Work out the finished part from the listing and answer in its coordinate system (mm). A direction names the side the tool comes from. Coordinates: 2 decimals unless noted, no trailing zeros. Order: outer loops, then holes, each group sorted by start corner. A loop starts at its lowest first (then second) coordinate and runs counter-clockwise, first axis right, second up. Notation, with made-up numbers: (61.25, 10) -> (106.25, 10) arc R27 cw to (106.25, 38) -> close; hole circle Ø10 at (7, 22.25). An arc over 180 degrees is marked (long way). Answer as CSV lines item,"result". Start each with the question number.
Item 1: Straight lines are drawn through the part: L1, parallel to Z at x = 44, y = 12; L2, parallel to Z at x = 0, y = -10; L3, parallel to X at y = 8, z = 2.5. For each, find the intervals that lie inside material, in ascending order.
Item 2: Section A-A (y = 12.7) is taken. Write down the section's boundary in (x, z).
Item 3: Section D-D (x = 44) is taken. Write down the section's boundary in (y, z) (3 decimals).
Item 4: Which of the six approach directions +Z, -Z, +X, -X, +Y, -Y give full straight-line access (tool end or side, diameter ignored) to faces 4 (the face through (1.4, 11.112, 18.2)), 5 (the face through (8.2, -4.763, -8.2)), 6 (the face through (31.75, -13, -16)), 7 (the face through (25, 0, 25.4))?
Item 5: Section C-C (x = 6) is taken. Write down the section's boundary in (y, z) (1 decimal), then the cut area to 3 significant figures.
Item 6: Each of these flat-tipped pins is pushed along its axis until it touches: pin 1 Ø2.5 at (x, z) = (10.78, -10.78) entering from -Y; pin 2 Ø4 at (x, y) = (-5, 13) entering from -Z; pin 3 Ø8 at (x, y) = (-11.5, -2) entering from +Z; pin 4 Ø2 at (x, z) = (-10.78, -10.78) entering from -Y. Where does it stop, or does it pass through?
Item 7: For a pull along Y with two mould halves and no side action, classify faces 1 (the face through (-15.12, -13.62, -11.59)), 2 (the face through (31.75, 13, 16)), 3 (the face through (21, 22.225, 0)) as pulls with the +Y half, pulls with the -Y half, needs draft (parallel to the pull), parting line crosses it, or undercut.
```python
from build123d import *

# Parameters (mm, degrees)
SKETCH1_W           = 76.2
SKETCH1_H           = 50.8
BOSS_EXTRUDE1_DEPTH = 22.225
SKETCH2_R           = 20.5994
CUT_EXTRUDE1_DEPTH  = 11.1125
SKETCH3_R           = 18.0975
CUT_EXTRUDE2_DEPTH  = 9.525
SKETCH4_R           = 9.6266
CUT_EXTRUDE3_DEPTH  = 24.8125
SKETCH5_R           = 19.05
CUT_EXTRUDE4_DEPTH  = 17.4625
SKETCH6_R           = 11.303
CUT_EXTRUDE5_DEPTH  = 1.397
SKETCH7_R           = 3.2639
CUT_EXTRUDE6_DEPTH  = 19.05
SKETCH8_R           = 1.1811
CUT_EXTRUDE7_DEPTH  = 27.9875
CIRPATTERN1_COUNT   = 4
CUT_EXTRUDE8_DEPTH  = 45.45


with BuildPart() as part:
    # Sketch1 → Boss-Extrude1 (new body, symmetric)
    with BuildSketch(Plane(origin=(0, 0, 0), x_dir=(1, 0, 0), z_dir=(0, 1, 0))):
        with Locations((12.7, 0)):
            Rectangle(SKETCH1_W, SKETCH1_H)
    extrude(amount=BOSS_EXTRUDE1_DEPTH, both=True)

    # Sketch2 → Cut-Extrude1 (cut)
    with BuildSketch(Plane(origin=(0, 22.225, 0), x_dir=(1, 0, 0), z_dir=(0, 1, 0))):
        Circle(SKETCH2_R)
    extrude(amount=-CUT_EXTRUDE1_DEPTH, mode=Mode.SUBTRACT)

    # Sketch3 → Cut-Extrude2 (cut)
    with BuildSketch(Plane(origin=(0, 11.1125, 0), x_dir=(1, 0, 0), z_dir=(0, 1, 0))):
        Circle(SKETCH3_R)
    extrude(amount=-CUT_EXTRUDE2_DEPTH, mode=Mode.SUBTRACT)

    # Sketch4 → Cut-Extrude3 (cut, through all)
    with BuildSketch(Plane(origin=(0, 1.5875, 0), x_dir=(1, 0, 0), z_dir=(0, 1, 0))):
        Circle(SKETCH4_R)
    extrude(amount=-CUT_EXTRUDE3_DEPTH, mode=Mode.SUBTRACT)

    # Sketch5 → Cut-Extrude4 (cut)
    with BuildSketch(Plane.XZ.offset(22.225)):
        Circle(SKETCH5_R)
    extrude(amount=-CUT_EXTRUDE4_DEPTH, mode=Mode.SUBTRACT)

    # Sketch6 → Cut-Extrude5 (cut)
    with BuildSketch(Plane.XZ.offset(4.7625)):
        Circle(SKETCH6_R)
    extrude(amount=-CUT_EXTRUDE5_DEPTH, mode=Mode.SUBTRACT)

    # Sketch7 → Cut-Extrude6 (cut)
    with BuildSketch(Plane(origin=(50.8, 0, 0), x_dir=(0, 0, -1), z_dir=(1, 0, 0))):
        with Locations((-15.875, 12.7)):
            Circle(SKETCH7_R)
        with Locations((15.875, 12.7)):
            Circle(SKETCH7_R)
        with Locations((-15.875, -12.7)):
            Circle(SKETCH7_R)
        with Locations((15.875, -12.7)):
            Circle(SKETCH7_R)
    extrude(amount=-CUT_EXTRUDE6_DEPTH, mode=Mode.SUBTRACT)

    # Sketch8 → Cut-Extrude7 (cut, through all)
    with BuildSketch(Plane.XZ.offset(4.7625)):
        with Locations((-10.776307345, 10.776307345)):
            Circle(SKETCH8_R)
    cut_extrude7 = extrude(amount=-CUT_EXTRUDE7_DEPTH, mode=Mode.SUBTRACT)

    # CirPattern1: Cut-Extrude7 ×4 about axis
    cirpattern1_axis = Axis((0, 0, 0), (0, 1, 0))
    for i in range(1, CIRPATTERN1_COUNT):
        add(cut_extrude7.rotate(cirpattern1_axis, i * 360 / CIRPATTERN1_COUNT), mode=Mode.SUBTRACT)

    # Sketch9 → Cut-Extrude8 (cut, through all)
    with BuildSketch(Plane.XZ.offset(22.225)):
        with BuildLine():
            Line((0, 25.4), (0, 38.1))
            Line((0, 38.1), (-38.1, 38.1))
            Line((-38.1, 38.1), (-38.1, -38.1))
            Line((-38.1, -38.1), (0, -38.1))
            Line((0, -38.1), (0, -25.4))
            ThreePointArc((0, -25.4), (-25.4, 0), (0, 25.4))
        make_face()
    extrude(amount=-CUT_EXTRUDE8_DEPTH, mode=Mode.SUBTRACT)


solid = part.part
```
Checked values:
1,L1,"z = -25.4 to -19.06, -12.69 to 12.69, 19.06 to 25.4"
1,L2,"z = -25.4 to -19.05, 19.05 to 25.4"
1,L3,"x = -25.28 to -17.92, 17.92 to 50.8"
2,outline,"(0, -25.4) -> (50.8, -25.4) -> (50.8, -19.14) -> (31.75, -19.14) -> (31.75, -12.61) -> (50.8, -12.61) -> (50.8, 12.61) -> (31.75, 12.61) -> (31.75, 19.14) -> (50.8, 19.14) -> (50.8, 25.4) -> (0, 25.4) arc R25.4 ccw to start; hole circle Ø41.2 at (0, 0)"
3,outline,"(-22.225, -25.4) -> (22.225, -25.4) -> (22.225, 25.4) -> (-22.225, 25.4) -> close; hole circle Ø6.528 at (-12.7, -15.875); hole circle Ø6.528 at (-12.7, 15.875); hole circle Ø6.528 at (12.7, -15.875); hole circle Ø6.528 at (12.7, 15.875)"
4,face 4,"+Y"
4,face 5,"-Y"
4,face 6,"+X"
4,face 7,"+Z, +X, -X, +Y, -Y"
5,outline,"(-22.2, -25.4) -> (22.2, -25.4) -> (22.2, -19.7) -> (11.1, -19.7) -> (11.1, -17.1) -> (1.6, -17.1) -> (1.6, -7.5) -> (-3.4, -7.5) -> (-3.4, -9.6) -> (-4.8, -9.6) -> (-4.8, -18.1) -> (-22.2, -18.1) -> close; (-22.2, 18.1) -> (-4.8, 18.1) -> (-4.8, 9.6) -> (-3.4, 9.6) -> (-3.4, 7.5) -> (1.6, 7.5) -> (1.6, 17.1) -> (11.1, 17.1) -> (11.1, 19.7) -> (22.2, 19.7) -> (22.2, 25.4) -> (-22.2, 25.4) -> close"
5,area,"762 mm^2"
6,pin 1,"stops at y = -4.76"
6,pin 2,"stops at z = -25.22"
6,pin 3,"stops at z = 24.27"
6,pin 4,"passes through"
7,face 1,"needs draft"
7,face 2,"undercut"
7,face 3,"pulls with the +Y half"
